Print and shaded views of the part. All mm, measured from the part's lowest x, y and z. A direction names the side the tool comes from. Round coordinates to 2 decimals unless told otherwise and drop trailing zeros. Order: outer loops, then holes, each group sorted by start corner. A loop starts at its lowest first (then second) coordinate and runs counter-clockwise, first axis right, second up. Notation, with made-up numbers: (62, -40) - (97, -40) arc R20 cw to (97, -18) - close; hole circle Ø1 at (82.25, 34). An arc over 180 degrees is marked (long way). Return JSON: item names as keys, results as strings. Group by question number.
Item 1: Two-plate mould, pull along Y, no slides. Class the marked faces 1, 2 and 3: released by +Y, released by -Y, zero draft, split by the parting line, or undercut.
Item 2: Saw through at C-C on y = 1.25. List the corners of the cut face in (x, z).
Item 3: Drop flat-ended pins along their axis: pin 1 (2 mm diameter, centred on x = 2.5, z = 2.5, fed in from -Y); pin 2 (4 mm diameter, centred on y = 9, z = 5, fed in from -X); pin 3 (5 mm diameter, centred on y = 4, z = 8, fed in from +X); pin 4 (3.5 mm diameter, centred on x = 5.5, z = 4.5, fed in from -Y). Give the stop position or say it passes through.
Item 4: Saw through at A-A on z = 5. List the corners of the cut face in (x, y).
Item 5: Tool access for the marked faces 4, 5 and 6: list every direction of +Z, -Z, +X, -X, +Y, -Y with a clear straight run to the whole face (end or side of a thin tool).
Item 6: Probe probe 1 along Y at (x, z) = (6.5, 4); probe 2 along Y at (x, z) = (7.5, 6); probe 3 along Y at (x, z) = (3.65, 5). List the from-to ranges inside material, lowest first.
Item 7: Saw through at B-B on y = 9. List the corners of the cut face in (x, z), and give its area (3 significant figures).
Item 8: Saw through at D-D on x = 7. State how many separate pieces and enclosed holes the cut face has, and give its area (3 significant figures).
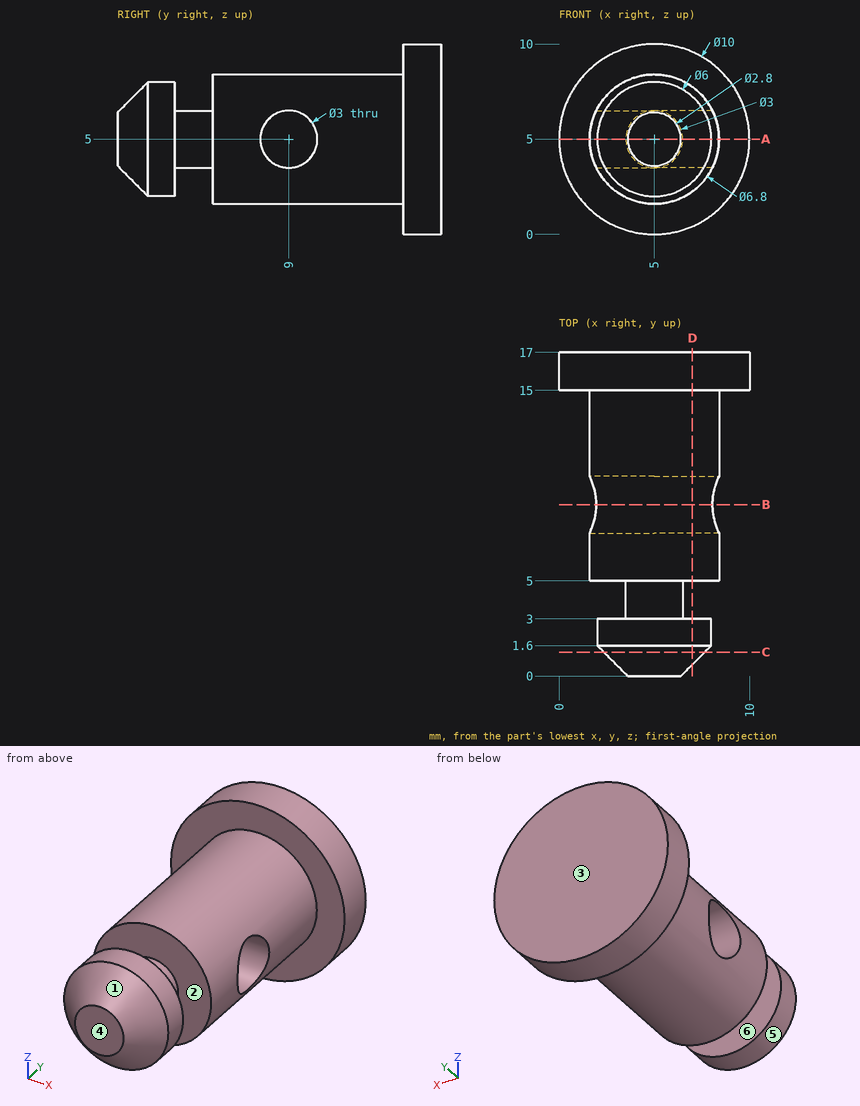
Filled in:
{
 "1": {"face 1": "released by -Y", "face 2": "undercut", "face 3": "released by +Y"},
 "2": {"outline": "circle Ø5.3 at (5, 5)"},
 "3": {"pin 1": "stops at y = 1.14", "pin 2": "stops at x = 1.6", "pin 3": "stops at x = 8.33", "pin 4": "stops at y = 0"},
 "4": {"outline": "(0, 15) - (1.6, 15) - (1.6, 10.5) - (8.4, 10.5) - (8.4, 15) - (10, 15) - (10, 17) - (0, 17) - close; (1.6, 5) - (3.5, 5) - (3.5, 3) - (2, 3) - (2, 1.6) - (3.6, 0) - (6.4, 0) - (8, 1.6) - (8, 3) - (6.5, 3) - (6.5, 5) - (8.4, 5) - (8.4, 7.5) - (1.6, 7.5) - close"},
 "5": {"face 4": "+Z, -Z, +X, -X, -Y", "face 5": "-Y", "face 6": "none"},
 "6": {"probe 1": "y = 0.4 to 3, 5 to 7.88, 10.12 to 17", "probe 2": "y = 1.29 to 3, 5 to 7.88, 10.12 to 17", "probe 3": "y = 0 to 7.5, 10.5 to 17"},
 "7": {"outline": "(1.95, 3.5) arc R3.4 ccw to (8.05, 3.5) - close; (1.95, 6.5) - (8.05, 6.5) arc R3.4 ccw to start", "area": "16.6 mm^2"},
 "8": {"separate pieces": "2", "enclosed holes": "1", "area": "75.4 mm^2"}
}
